Here's how the part is built. I have some questions about the finished solid (model axes, mm). Face numbers are marked on the shaded views. A direction names the side the tool comes from. Give positions to 0.01 mm unless a question says otherwise; leave off trailing zeros. Write each loop counter-clockwise with the first axis right and the second up, starting at its lowest first coordinate (ties: lowest second). Pieces come first, ordered by that corner, then holes. Notation, with made-up numbers: (10.25, 89.25) - (69.25, 89.25) arc R28 ccw to (69.25, 113.25) - close; hole circle Ø5 at (35.5, 9.5). An arc over 180 degrees is marked (long way). One line per item, written item: value. Start each with the question number.
1) I'm going to push flat-ended pins straight in: P1, Ø20.5, axis at x = -27, z = 146, coming from the +Y side; P2, Ø1, axis at x = 34.5, y = 3, coming from the +Z side; P3, Ø9.5, axis at x = -24.5, z = 134, coming from the -Y side. Where does each tip first touch, or does it pass through?
2) Imagine slicing it at C-C on x = -50. Write out the boundary of the cut face in (y, z), plus the area to 3 significant figures.
3) Imagine slicing it at B-B on y = 6. Write out the boundary of the cut face in (x, z), plus the area to 3 significant figures.
4) On a 3-axis mill with a long thin cutter (end or side, diameter ignored), from which of +Z, -Z, +X, -X, +Y, -Y can I reach the whole of each face in a straight line? I mean the marked faces 1, 2, 3 and 4. Say none if no direction works.
5) Please list where these lines run through material, in increasing order: L1, parallel to Z at x = -53, y = 13.5; L2, parallel to Z at x = -3, y = -10.5; L3, parallel to Y at x = 32.5, z = 117.5. Write a range as [from, to].
from build123d import *

# Parameters (mm, degrees)
F0_R       = 16.5
F1_DEPTH   = 80
F2_W       = 140
F2_H       = 35
F2_R       = 16.5
F3_DEPTH   = 15
F4_W       = 70
F4_H       = 27.5
F5_DEPTH   = 360
F7_DEPTH   = 50
F8_SIZE2   = 13.75
F8_SIZE    = 51.3156986041
F8_2_SIZE2 = 13.74999
F8_2_SIZE  = 51.315689


# Not quite as in the source:
# - a fillet or chamfer is up to 0.001 mm smaller than in the source, because OpenCascade refuses the exact size


with BuildPart() as f1:
    # F0 (on Top) → F1 (new body)
    with BuildSketch(Plane.XY):
        Circle(F0_R)
    extrude(amount=-F1_DEPTH)

    # F2 (on face) → F3 (join)
    with BuildSketch(Plane.XY):
        Rectangle(F2_W, F2_H)
        Circle(F2_R, mode=Mode.SUBTRACT)
    extrude(amount=-F3_DEPTH)

    # F4 (on face) → F5 (join)
    with BuildSketch(Plane.XY):
        Rectangle(F4_W, F4_H)
    extrude(amount=F5_DEPTH)

    # F6 (on face) → F7 (cut)
    with BuildSketch(Plane.XZ.offset(13.75)):
        Polygon((35, 360), (-35, 360), (35, 279.5273661613), align=None)
    extrude(amount=-F7_DEPTH, mode=Mode.SUBTRACT)

    # F8
    f8_edges = [f1.edges().sort_by_distance(p)[0] for p in [
        (35, 13.75, 139.763683),
        (0, 13.75, 319.763683),
    ]]
    f8_side = f1.faces().sort_by_distance((-1.468033, 13.75, 160.725674))[0]
    chamfer(f8_edges, length=F8_SIZE, length2=F8_SIZE2, reference=f8_side)

    # F8#2 (size 51.3156986041 and 13.75 in the source; OpenCascade refuses exactly that, so slightly less here)
    f8_2_edges = [f1.edges().sort_by_distance(p)[0] for p in [
        (35, -13.75, 139.763683),
        (0, -13.75, 319.763683),
    ]]
    f8_2_side = f1.faces().sort_by_distance((-1.468033, -13.75, 160.725674))[0]
    chamfer(f8_2_edges, length=F8_2_SIZE, length2=F8_2_SIZE2, reference=f8_2_side)


solid = f1.part
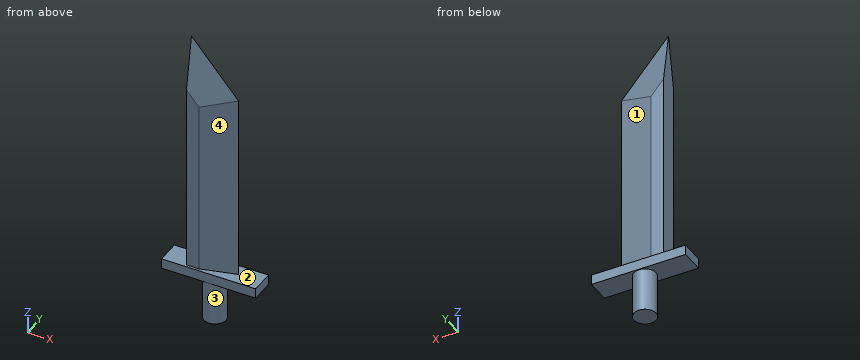
Numbers:
1. P1: y = 13.75
1. P2: z = 0
1. P3: y = -13.75
2. outline: (-17.5, -15) - (17.5, -15) - (17.5, 0) - (-17.5, 0) - close
2. area: 525 mm^2
3. outline: (-70, -15) - (-15.37, -15) - (-15.37, -80) - (15.37, -80) - (15.37, -15) - (70, -15) - (70, 0) - (12.61, 0) - (12.61, 271.15) - (-35, 325.88) - (-35, 0) - (-70, 0) - close
3. area: 18,300 mm^2
4. face 1: +Z, +X, +Y
4. face 2: +Z
4. face 3: -Z
4. face 4: +Z, +X, -Y
5. L1: [-15, 0]
5. L2: [-80, 0]
5. L3: [-0.67, 0.67]
